```python
from build123d import *

# Parameters (mm, degrees)
F1_DEPTH = 2300
F2_R     = 5
F3_R     = 5


with BuildPart() as f1:
    # F0 (on Right) → F1 (new body)
    with BuildSketch(Plane.YZ):
        with BuildLine():
            ThreePointArc((109.3978564406, 919.1393998067), (106.0671493896, 917.2549764252), (105.0444723994, 913.5673223315))
            Line((105.0444723994, 913.5673223315), (153.0993439735, 522.1918006805))
            ThreePointArc((153.0993439735, 522.1918006805), (154.983767355, 518.8610936295), (158.6714214487, 517.8384166393))
            Line((158.6714214487, 517.8384166393), (186.0489625337, 521.199956))
            ThreePointArc((186.0489625337, 521.199956), (189.3796695847, 523.0843793816), (190.4023465749, 526.7720334753))
            Line((190.4023465749, 526.7720334753), (142.3474750008, 918.1475551263))
            ThreePointArc((142.3474750008, 918.1475551263), (140.4630516192, 921.4782621773), (136.7753975256, 922.5009391675))
            Line((136.7753975256, 922.5009391675), (109.3978564406, 919.1393998067))
        make_face()
    extrude(amount=-F1_DEPTH)

    # F2
    f2_edges = [f1.edges().sort_by_distance(p)[0] for p in [
        (0, 140.463052, 921.478262),
        (0, 123.086627, 920.820169),
        (0, 106.067149, 917.254976),
        (0, 129.071908, 717.879562),
        (0, 154.983767, 518.861094),
        (0, 172.360192, 519.519186),
        (0, 189.37967, 523.084379),
        (0, 166.374911, 722.459794),
    ]]
    fillet(f2_edges, radius=F2_R)

    # F3
    f3_edges = [f1.edges().sort_by_distance(p)[0] for p in [
        (-2300, 140.463052, 921.478262),
        (-2300, 123.086627, 920.820169),
        (-2300, 106.067149, 917.254976),
        (-2300, 129.071908, 717.879562),
        (-2300, 154.983767, 518.861094),
        (-2300, 172.360192, 519.519186),
        (-2300, 189.37967, 523.084379),
        (-2300, 166.374911, 722.459794),
    ]]
    fillet(f3_edges, radius=F3_R)


solid = f1.part
```
Work out the finished part from the listing and answer in its coordinate system (mm). Give positions to 0.01 mm unless a question says otherwise; leave off trailing zeros. Order: outer loops, then holes, each group sorted by start corner. A loop starts at its lowest first (then second) coordinate and runs counter-clockwise, first axis right, second up. Notation, with made-up numbers: (-0.75, 1.5) -> (15.25, 1.5) arc R16 cw to (15.25, 13.5) -> close; hole circle Ø9 at (-12.5, 36). An arc over 180 degrees is marked (long way). Answer as CSV lines item,"result". Start each with the question number.
(1) Section A-A, the plane x = -2037 is taken. Write down the section's boundary in (y, z), plus the area to 3 significant figures.
(2) Each of these flat-tipped pins is pushed along its axis until it touches: pin 1 Ø6 at (x, z) = (-1372, 672.5) entering from -Y; pin 2 Ø6 at (x, z) = (-1636, 805) entering from -Y; pin 3 Ø10 at (x, z) = (-708.5, 605) entering from -Y. Where does it stop, or does it pass through?
(3) Consider line 1 along Y through (x, z) = (-467.5, 729.5); line 2 along Y through (x, z) = (-1055, 831.5); line 3 along X through (y, z) = (118, 826). Determine where each line is inside the solid, lowest interval first.
Entries:
1,outline,"(105.04, 913.57) -> (153.1, 522.19) arc R5 ccw to (158.67, 517.84) -> (186.05, 521.2) arc R5 ccw to (190.4, 526.77) -> (142.35, 918.15) arc R5 ccw to (136.78, 922.5) -> (109.4, 919.14) arc R5 ccw to start"
1,area,"15,200 mm²"
2,pin 1,"y = 134.28"
2,pin 2,"y = 118.01"
2,pin 3,"y = 142.32"
3,line 1,"127.65 to 165.51"
3,line 2,"115.12 to 152.99"
3,line 3,"-2299.13 to -0.87"
